Geometry: final body of the model. Coordinates: model frame, mm. Round coordinates to 2 decimals unless told otherwise and drop trailing zeros. Loops run counter-clockwise (first coordinate to the right, second up) from the corner with the lowest first, then second, coordinate; pieces in that order, holes last. Notation, with made-up numbers: (-13.75, 5) - (28.25, 5) arc R29 ccw to (28.25, 36) - close; hole circle Ø4 at (31.25, 80.5). An arc over 180 degrees is marked (long way). Write item = value, one per line. Start each with the question number.
Item 1: First-contact query: pin 1 (1.1 mm diameter, centred on y = 5.5, z = 125.5, fed in from -X); pin 2 (1.9 mm diameter, centred on y = 6, z = 81, fed in from +X); pin 3 (5 mm diameter, centred on x = 8.5, z = 202, fed in from -Y). Flat tips, straight axial feed; report the tip coordinate or a pass-through.
Item 2: Section A-A (y = 2.75). Return loops of the section in (x, z), plus the area to 3 significant figures.
Item 3: Line query: line 1 (Z direction, x = 8.5, y = 6.5); line 2 (X direction, y = 7.1, z = 202); line 3 (Z direction, x = 9.75, y = 4.75). Output: solid intervals per line, ascending. Write a range as from..to.
Item 4: Section B-B (z = 69). Return loops of the section in (x, y).
Autodesk Inventor part; units mm, degrees
ref_plane "YZ Plane" through (0, 0, 0) normal (1, 0, 0) x (0, 1, 0)
ref_plane "XZ Plane" through (0, 0, 0) normal (0, 1, 0) x (-1, 0, 0)
ref_plane "XY Plane" through (0, 0, 0) normal (0, 0, 1) x (1, 0, 0)
sketch "スケッチ1" plane through (0, 0, 0) normal (0, 0, 1) x (1, 0, 0)
  line L0 (0, 0) -> (16.2361, 0)
  line L1 (17, 8) -> (0, 8)
  line L2 (3, 0) -> (14, 0)
  line L3 (14, 0) -> (14, 4)
  line L4 (14, 4) -> (3, 4)
  line L5 (3, 4) -> (3, 0)
  arc A0 (16.2361, 0) -> (16, 4.2361) centre (14, 2) ccw
  arc A1 (1, 4.2361) -> (0.7639, 0) centre (3, 2) ccw
  line L6 (16, 8) -> (16, 4.2361)
  line L7 (1, 8) -> (1, 4.2361)
  point P0 (8.5, 8)
  point P1 (8.5, 4)
  dimension "d0" = 17
  dimension "d2" = 11
  dimension "d3" = 4
  dimension "d15" = 7.5
  dimension "d16" = 15
  dimension "d17" = 8
  dimension "d18" = 17
extrude "押し出し1" add sketch "スケッチ1" along normal blind 246 contours A1 L7 L1 L6 A0 L0 L3 L4 L5
sketch "スケッチ2" plane through (0, 8, 0) normal (0, 1, 0) x (1, 0, 0)
  line L0 (16, 0) -> (0, 0)
  line L1 (-88, 0) -> (-88, -156.2142)
  line L2 (-88, -156.2142) -> (215.5, -300.2142)
  line L3 (3, 0) -> (3, -246)
  point P0 (8.5, -5)
  point P1 (8.5, -202)
  point P2 (8, 0)
  point P3 (17, 0)
  point P4 (1, 0)
  dimension "d6" = 5
  dimension "d20" = 96
  dimension "d21" = 303.5
  dimension "d22" = 144
  dimension "d23" = 5.5
  dimension "d24" = 197
hole "穴1" at (8.5, 8, 5) at (8.5, 8, 202) direction (0, -1, 0) diameter 3 depth 8 tip angle 118
properties part number "slider4b"
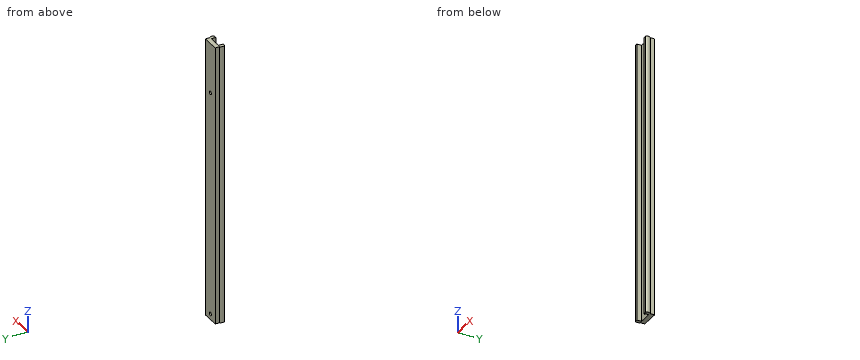
Taken from the geometry:
q1.pin_1 = 1
q1.pin_2 = 16
q1.pin_3 = 4
q2.outline = (0.1, 0) - (3, 0) - (3, 246) - (0.1, 246) - close; (14, 0) - (16.9, 0) - (16.9, 246) - (14, 246) - close
q2.area = 1,430 mm^2
q3.line_1 = 0..3.5, 6.5..200.5, 203.5..246
q3.line_2 = 1..7, 10..16
q3.line_3 = 0..4.17, 5.83..201.17, 202.83..246
q4.outline = (0.76, 0) - (3, 0) - (3, 4) - (14, 4) - (14, 0) - (16.24, 0) arc R3 ccw to (16, 4.24) - (16, 8) - (1, 8) - (1, 4.24) arc R3 ccw to start
